```python
from build123d import *

# Parameters (mm, degrees)
F0_W     = 101.6
F0_H     = 50.8
F1_DEPTH = 25.4
F2_W     = 101.6
F2_H     = 38.1
F3_DEPTH = 50.8
F4_W     = 50.8
F4_H     = 38.1
F5_DEPTH = 19.05


with BuildPart() as f1:
    # F0 (on Top) → F1 (new body)
    with BuildSketch(Plane.XY):
        with Locations((25.266851, 12.138548)):
            Rectangle(F0_W, F0_H)
    extrude(amount=F1_DEPTH)

    # F2 (on face) → F3 (join)
    with BuildSketch(Plane.XY.offset(25.4)):
        with Locations((25.266851, 18.488548)):
            Rectangle(F2_W, F2_H)
    extrude(amount=F3_DEPTH)

    # F4 (on face) → F5 (cut)
    with BuildSketch(Plane.XZ.offset(0.561452)):
        with Locations((25.266851, 57.15)):
            Rectangle(F4_W, F4_H)
    extrude(amount=-F5_DEPTH, mode=Mode.SUBTRACT)


solid = f1.part
```
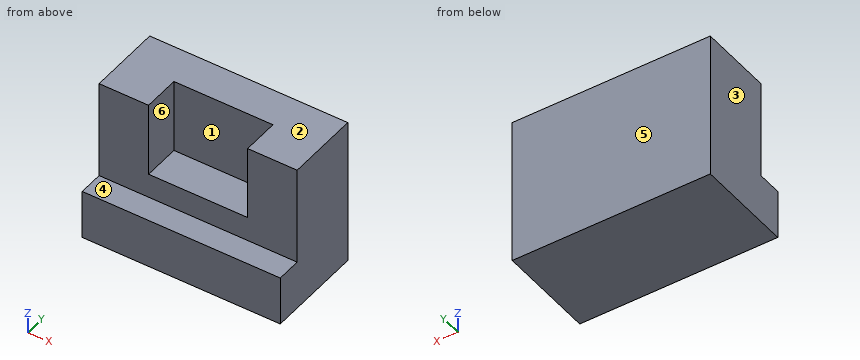
Work out the finished part from the listing and answer in its coordinate system (mm). Face numbers are marked on the shaded views. A direction names the side the tool comes from. Give positions to 0.01 mm unless a question says otherwise; leave off trailing zeros. Write each loop counter-clockwise with the first axis right and the second up, starting at its lowest first coordinate (ties: lowest second). Pieces come first, ordered by that corner, then holes. Notation, with made-up numbers: (9.5, 62.25) -> (34.5, 62.25) arc R4 ccw to (34.5, 68.25) -> close; hole circle Ø4 at (-38.5, 54.25). An arc over 180 degrees is marked (long way). Write item = value, one per line.
Q1. Consider line 1 along X through (y, z) = (1, 39); line 2 along Y through (x, z) = (-12.5, 49.5); line 3 along Y through (x, z) = (14, 55). Determine where each line is inside the solid, lowest interval first.
Computed values:
line_1 = -25.53 to -0.13, 50.67 to 76.07
line_2 = -0.56 to 37.54
line_3 = 18.49 to 37.54
Q2. For a pull along X with two mould halves and no side action, classify the marked faces 1, 2 and 3 as pulls with the +X half, pulls with the -X half, needs draft (parallel to the pull), parting line crosses it, or undercut.
Computed values:
face_1 = undercut
face_2 = needs draft
face_3 = pulls with the -X half
Q3. Section C-C on x = -5 is taken. Determine the outline of the cut face in (y, z), and give its area (3 significant figures).
Computed values:
outline = (-13.26, 0) -> (37.54, 0) -> (37.54, 76.2) -> (-0.56, 76.2) -> (-0.56, 25.4) -> (-13.26, 25.4) -> close
area = 3,230 mm^2
Q4. Section A-A on y = 9 is taken. Determine the outline of the cut face in (x, z).
Computed values:
outline = (-25.53, 0) -> (76.07, 0) -> (76.07, 76.2) -> (50.67, 76.2) -> (50.67, 38.1) -> (-0.13, 38.1) -> (-0.13, 76.2) -> (-25.53, 76.2) -> close
Q5. A tool of negligible diameter and unlimited length cuts with its end or side. For the marked faces 4, 5 and 6, from which of +Z, -Z, +X, -X, +Y, -Y can it reach the whole face along a straight path? Write none if from no direction.
Computed values:
face_4 = +Z, +X, -X, -Y
face_5 = +Z, -Z, +X, -X, +Y
face_6 = +Z, -Y
Q6. Section D-D on y = -8.5 is taken. Determine the outline of the cut face in (x, z).
Computed values:
outline = (-25.53, 0) -> (76.07, 0) -> (76.07, 25.4) -> (-25.53, 25.4) -> close
Q7. Section B-B on z = 47 is taken. Determine the outline of the cut face in (x, y).
Computed values:
outline = (-25.53, -0.56) -> (-0.13, -0.56) -> (-0.13, 18.49) -> (50.67, 18.49) -> (50.67, -0.56) -> (76.07, -0.56) -> (76.07, 37.54) -> (-25.53, 37.54) -> close
Q8. Flat-ended cylindrical pins translate along their axes: pin 1 Ø1 at (x, y) = (11.5, -1) entering from -Z; pin 2 Ø5 at (x, z) = (28, 57.5) entering from -Y; pin 3 Ø4 at (x, y) = (5.5, -7) entering from +Z; pin 4 Ø4 at (x, z) = (-2.5, 29.5) entering from -Y. Find the tip coordinate at first contact, or state that the pin passes through.
Computed values:
pin_1 = 0
pin_2 = 18.49
pin_3 = 25.4
pin_4 = -0.56
